Design review of the part built by this model. Coordinates are the model's own, in mm. A direction names the side the tool comes from. Coordinates: 2 decimals unless noted, no trailing zeros. Write each loop counter-clockwise with the first axis right and the second up, starting at its lowest first coordinate (ties: lowest second). Pieces come first, ordered by that corner, then holes.
```python
from build123d import *

# Parameters (mm, degrees)
BOSS_EXTRUDE1_DEPTH  = 10
CUT_EXTRUDE1_DEPTH   = 3
FILLET1_R            = 2
FILLET1_OF_MIRROR1_R = 2
SKETCH3_R            = 15
SKETCH3_R_2          = 14
CUT_EXTRUDE2_DEPTH   = 6
SKETCH3_3_R          = 14
CUT_EXTRUDE3_DEPTH   = 14
SKETCH3_4_R          = 6.5
CUT_EXTRUDE4_DEPTH   = 154.430766146
SKETCH4_R            = 5
CUT_EXTRUDE5_DEPTH   = 20
FILLET2_R            = 5


with BuildPart() as part:
    # Sketch1 → Boss-Extrude1 (new, symmetric)
    with BuildSketch(Plane(origin=(0, 0, 0), x_dir=(0, 0, -1), z_dir=(1, 0, 0))):
        with BuildLine():
            Line((-16, 137), (-26, 137))
            Line((-26, 137), (-30, 133))
            Line((-30, 133), (-30, 86.06334964))
            ThreePointArc((-30, 86.06334964), (-30.363636327, 80.044097084), (-31.449256053, 74.112397284))
            Line((-31.449256053, 74.112397284), (-46, 15))
            Line((-46, 15), (-46, 0))
            Line((-46, 0), (46, 0))
            Line((46, 0), (46, 15))
            Line((46, 15), (31.449256053, 74.112397284))
            ThreePointArc((31.449256053, 74.112397284), (30.363636327, 80.044097084), (30, 86.06334964))
            Line((30, 86.06334964), (30, 133))
            Line((30, 133), (26, 137))
            Line((26, 137), (16, 137))
            ThreePointArc((16, 137), (0, 145), (-16, 137))
        make_face()
    extrude(amount=BOSS_EXTRUDE1_DEPTH, both=True)

    # Sketch2 → Cut-Extrude1 (cut)
    with BuildSketch(Plane(origin=(10, 0, 0), x_dir=(0, 0, -1), z_dir=(1, 0, 0))):
        with BuildLine():
            Line((13, 100), (-13, 100))
            ThreePointArc((-13, 100), (-16.535533906, 98.535533906), (-18, 95))
            Line((-18, 95), (-18, 78.544796086))
            Line((-18, 78.544796086), (-30.886080209, 26.195095236))
            ThreePointArc((-30.886080209, 26.195095236), (-29.966452179, 21.915804495), (-26.031005815, 20))
            Line((-26.031005815, 20), (26.031005815, 20))
            ThreePointArc((26.031005815, 20), (29.966452179, 21.915804495), (30.886080209, 26.195095236))
            Line((30.886080209, 26.195095236), (18, 78.544796086))
            Line((18, 78.544796086), (18, 95))
            ThreePointArc((18, 95), (16.535533906, 98.535533906), (13, 100))
        make_face()
    cut_extrude1 = extrude(amount=-CUT_EXTRUDE1_DEPTH, mode=Mode.SUBTRACT)

    # Fillet1
    fillet1_edges = [part.edges().sort_by_distance(p)[0] for p in [
        (7, 52.369945661, 24.443040105),
        (7, 86.772398043, 18),
        (7, 98.535533906, 16.535533906),
        (7, 100, 0),
        (7, 98.535533906, -16.535533906),
        (7, 86.772398043, -18),
        (7, 52.369945661, -24.443040105),
        (7, 21.915804495, -29.966452179),
        (7, 20, 0),
        (7, 21.915804495, 29.966452179),
    ]]
    fillet(fillet1_edges, radius=FILLET1_R)

    # Mirror1: Cut-Extrude1 across plane
    add(cut_extrude1.mirror(Plane(origin=(0, 0, 0), x_dir=(0, 0, 1), z_dir=(1, 0, 0))), mode=Mode.SUBTRACT)

    # Fillet1 of Mirror1
    fillet1_of_mirror1_edges = [part.edges().sort_by_distance(p)[0] for p in [
        (-7, 52.369945661, 24.443040105),
        (-7, 86.772398043, 18),
        (-7, 98.535533906, 16.535533906),
        (-7, 100, 0),
        (-7, 98.535533906, -16.535533906),
        (-7, 86.772398043, -18),
        (-7, 52.369945661, -24.443040105),
        (-7, 21.915804495, -29.966452179),
        (-7, 20, 0),
        (-7, 21.915804495, 29.966452179),
    ]]
    fillet(fillet1_of_mirror1_edges, radius=FILLET1_OF_MIRROR1_R)

    # Sketch3 → Cut-Extrude2 (cut)
    with BuildSketch(Plane(origin=(10, 0, 0), x_dir=(0, 0, -1), z_dir=(1, 0, 0))):
        with Locations((0, 125)):
            Circle(SKETCH3_R)
        with Locations((0, 125)):
            Circle(SKETCH3_R_2, mode=Mode.SUBTRACT)
    extrude(amount=-CUT_EXTRUDE2_DEPTH, mode=Mode.SUBTRACT)

    # Sketch3_3 → Cut-Extrude3 (cut)
    with BuildSketch(Plane(origin=(10, 0, 0), x_dir=(0, 0, -1), z_dir=(1, 0, 0))):
        with Locations((0, 125)):
            Circle(SKETCH3_3_R)
    extrude(amount=-CUT_EXTRUDE3_DEPTH, mode=Mode.SUBTRACT)

    # Sketch3_4 → Cut-Extrude4 (cut, through all)
    with BuildSketch(Plane(origin=(10, 0, 0), x_dir=(0, 0, -1), z_dir=(1, 0, 0))):
        with Locations((0, 125)):
            Circle(SKETCH3_4_R)
    extrude(amount=-CUT_EXTRUDE4_DEPTH, mode=Mode.SUBTRACT)

    # Sketch4 → Cut-Extrude5 (cut)
    with BuildSketch(Plane.XZ):
        with Locations(Location((0, 30, 0), (0, 0, 270))):
            Circle(SKETCH4_R)
        with Locations(Location((0, -30, 0), (0, 0, 270))):
            Circle(SKETCH4_R)
    extrude(amount=-CUT_EXTRUDE5_DEPTH, mode=Mode.SUBTRACT)

    # Fillet2
    fillet2_edges = [part.edges().sort_by_distance(p)[0] for p in [
        (0, 137, 16),
        (0, 137, -16),
    ]]
    fillet(fillet2_edges, radius=FILLET2_R)


solid = part.part
```
(1) Consider section D-D (z = 10.5). Give the boundary of the cut face in (x, y), plus the area to 3 significant figures.
(2) Consider section C-C (x = 0). Give the boundary of the cut face in (y, z), plus the area to 3 significant figures.
(3) Insertion check: pin 1 Ø1.5 at (y, z) = (49, -16.5) entering from -X; pin 2 Ø0.8 at (x, y) = (-9.5, 90) entering from +Z; pin 3 Ø0.5 at (x, y) = (-9.5, 89) entering from -Z. Each pin has a flat end and moves straight along its axis. Give the tip position at first contact, or say it passes through.
(4) Wall thickness on line 1 (Y direction, x = 8.85, z = 0); line 2 (Y direction, x = -6.6, z = 0); line 3 (X direction, y = 14, z = -30): over which ranges is each line inside the solid? List them lowest first.
(5) Mouldability with a two-part tool opening along Z and no side actions: class faces 1 (the cylindrical face through (-0.14, 137.406, 16.357)), 2 (the flat face through (0, 109, -30)), 3 (the cylindrical face through (-7.6, 52.72, -23.77)), 4 (the cylindrical face through (9.51, 98.5, -16.57)) as +Z half, -Z half, draft (parallel to the pull), parting line (faces both ways), or undercut.
(6) Consider section B-B (z = 0). Give the boundary of the cut face in (x, y), plus the area to 3 significant figures.
(7) Consider section A-A (y = 125). Give the boundary of the cut face in (x, z), plus the area to 3 significant figures.
(8) For faces 5 (the flat face through (7, 52, 0)), 6 (the cylindrical face through (0.14, 80.128, 30.354)), 7 (the cylindrical face through (0, 145, 0)), 8 (the flat face through (-9.51, 52.74, 24.35)), 9 (the flat face through (0, 20, -30)), list the 3-axis set-ups (+Z, -Z, +X, -X, +Y, -Y) from which the entire face can be reached by the end or side of a thin tool; tool diameter is ignored.
Results:
1. outline: (-10, 0) - (10, 0) - (10, 20) - (9, 20) arc R2 cw to (7, 22) - (7, 98) arc R2 cw to (9, 100) - (10, 100) - (10, 114.29) - (4, 114.29) - (4, 115.74) - (-4, 115.74) - (-4, 134.26) - (4, 134.26) - (4, 135.71) - (10, 135.71) - (10, 142.02) - (-10, 142.02) - (-10, 100) - (-9, 100) arc R2 cw to (-7, 98) - (-7, 22) arc R2 cw to (-9, 20) - (-10, 20) - close
1. area: 2,090 mm2
2. outline: (0, -46) - (15, -46) - (74.11, -31.45) arc R50 cw to (86.06, -30) - (133, -30) - (137, -26) - (137, -18.33) arc R5 cw to (138.6, -14.66) arc R20 ccw to (138.6, 14.66) arc R5 cw to (137, 18.33) - (137, 26) - (133, 30) - (86.06, 30) arc R50 cw to (74.11, 31.45) - (15, 46) - (0, 46) - (0, 35) - (20, 35) - (20, 25) - (0, 25) - (0, -25) - (20, -25) - (20, -35) - (0, -35) - close; hole circle Ø28 at (125, 0)
2. area: 8,890 mm2
3. pin 1: stops at x = -7
3. pin 2: stops at z = 30
3. pin 3: stops at z = -30
4. line 1: y = 0 to 20.01, 99.99 to 110, 140 to 145
4. line 2: y = 0 to 118.5, 131.5 to 145
4. line 3: x = -10 to -5, 5 to 10
5. face 1: +Z half
5. face 2: -Z half
5. face 3: undercut
5. face 4: undercut
6. outline: (-10, 0) - (10, 0) - (10, 20) - (9, 20) arc R2 cw to (7, 22) - (7, 98) arc R2 cw to (9, 100) - (10, 100) - (10, 110) - (4, 110) - (4, 111) - (-4, 111) - (-4, 118.5) - (-10, 118.5) - (-10, 100) - (-9, 100) arc R2 cw to (-7, 98) - (-7, 22) arc R2 cw to (-9, 20) - (-10, 20) - close; (-10, 131.5) - (-4, 131.5) - (-4, 139) - (4, 139) - (4, 140) - (10, 140) - (10, 145) - (-10, 145) - close
6. area: 1,940 mm2
7. outline: (-10, -30) - (10, -30) - (10, -15) - (4, -15) - (4, -14) - (-4, -14) - (-4, -6.5) - (-10, -6.5) - close; (-10, 6.5) - (-4, 6.5) - (-4, 14) - (4, 14) - (4, 15) - (10, 15) - (10, 30) - (-10, 30) - close
7. area: 718 mm2
8. face 5: +X
8. face 6: +Z, +X, -X, +Y
8. face 7: +X, -X, +Y
8. face 8: -X
8. face 9: -Y
